Geometry: see drawing. Coordinates: mm, zero at the bounding-box minimum. Coordinates: 2 decimals unless noted, no trailing zeros. Write each loop counter-clockwise with the first axis right and the second up, starting at its lowest first coordinate (ties: lowest second). Pieces come first, ordered by that corner, then holes. Notation, with made-up numbers: (18.5, 1.25) -> (58.5, 1.25) arc R28 cw to (58.5, 31.25) -> close; hole circle Ø9 at (-40, 48). An arc over 180 degrees is marked (long way). Answer as a JSON object with one key per item and string values. Group by question number.
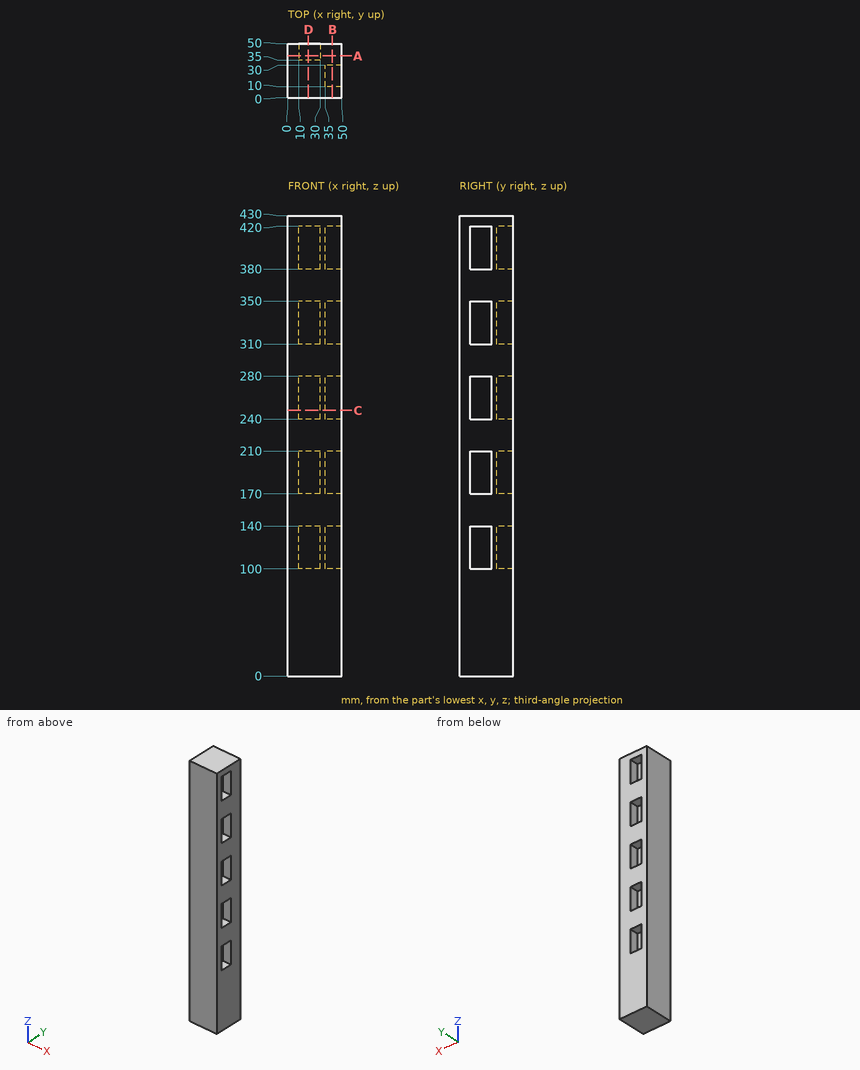
Item 1: Section C-C on z = 248. Output: boundary loops of the cut face in (x, y), then the cut area to 3 significant figures.
Item 2: Section A-A on y = 39. Output: boundary loops of the cut face in (x, z), then the cut area to 3 significant figures.
Item 3: Ray query, L1, parallel to Z at x = 25, y = 42; L2, parallel to Y at x = 45, z = 338. Return the intervals inside material, ascending. Write a range as [from, to].
Item 4: Section D-D on x = 19. Output: boundary loops of the cut face in (y, z).
Item 5: Contact query for flat-ended pins moving along their axis: pin 1 (10 mm diameter, centred on x = 18.5, z = 399.5, fed in from +Y); pin 2 (10 mm diameter, centred on y = 20, z = 336, fed in from +X). Output: stop coordinate, or through.
Answer sheet:
{
 "1": {"outline": "(0, 0) -> (50, 0) -> (50, 10) -> (35, 10) -> (35, 30) -> (50, 30) -> (50, 50) -> (30, 50) -> (30, 35) -> (10, 35) -> (10, 50) -> (0, 50) -> close", "area": "1,900 mm^2"},
 "2": {"outline": "(0, 0) -> (50, 0) -> (50, 430) -> (0, 430) -> close; hole (10, 100) -> (30, 100) -> (30, 140) -> (10, 140) -> close; hole (10, 170) -> (30, 170) -> (30, 210) -> (10, 210) -> close; hole (10, 240) -> (30, 240) -> (30, 280) -> (10, 280) -> close; hole (10, 310) -> (30, 310) -> (30, 350) -> (10, 350) -> close; hole (10, 380) -> (30, 380) -> (30, 420) -> (10, 420) -> close", "area": "17,500 mm^2"},
 "3": {"L1": "z = [0, 100], [140, 170], [210, 240], [280, 310], [350, 380], [420, 430]", "L2": "y = [0, 10], [30, 50]"},
 "4": {"outline": "(0, 0) -> (50, 0) -> (50, 100) -> (35, 100) -> (35, 140) -> (50, 140) -> (50, 170) -> (35, 170) -> (35, 210) -> (50, 210) -> (50, 240) -> (35, 240) -> (35, 280) -> (50, 280) -> (50, 310) -> (35, 310) -> (35, 350) -> (50, 350) -> (50, 380) -> (35, 380) -> (35, 420) -> (50, 420) -> (50, 430) -> (0, 430) -> close"},
 "5": {"pin 1": "stops at y = 35", "pin 2": "stops at x = 35"}
}
